from build123d import *

# Parameters (mm, degrees)
F1_DEPTH = 63.5
F2_DEPTH = 25.4
F3_DEPTH = 7.9375


with BuildPart() as f1:
    # F0 (on Front) → F1 (new body, symmetric)
    with BuildSketch(Plane.XZ):
        Polygon((22.225, 9.525), (-41.275, 9.525), (-41.275, -9.525), (41.275, -9.525), (41.275, 9.525), align=None)
    extrude(amount=F1_DEPTH, both=True)

    # F0 (on Front) → F2 (join, symmetric)
    with BuildSketch(Plane.XZ):
        with BuildLine():
            Line((22.225, 27.0002), (22.225, 9.525))
            Line((22.225, 9.525), (41.275, 9.525))
            Line((41.275, 9.525), (41.275, 27.0002))
            ThreePointArc((41.275, 27.0002), (45.92468, 38.22552), (57.15, 42.8752))
            Line((57.15, 42.8752), (67.710114, 42.8752))
            Line((67.710114, 42.8752), (67.710114, 61.9252))
            Line((67.710114, 61.9252), (57.15, 61.9252))
            add(Edge.make_bspline(
                [(56.676443, 61.921989), (56.834171, 61.923134), (56.992024, 61.924204), (57.15, 61.9252)],
                knots=[111.196311, 111.196311, 111.196311, 111.196311, 111.504536, 111.504536, 111.504536, 111.504536], degree=3))
            ThreePointArc((56.676443, 61.921989), (32.287432, 51.527905), (22.225, 27.0002))
        make_face()
    extrude(amount=F2_DEPTH, both=True)

    # F0 (on Front) → F3 (join, symmetric)
    with BuildSketch(Plane.XZ):
        with BuildLine():
            add(Edge.make_bspline(
                [(-41.275, 9.525), (-40.923248, 51.417116), (-0.225928, 61.509118), (56.676443, 61.921989)],
                knots=[0, 0, 0, 0, 111.196311, 111.196311, 111.196311, 111.196311], degree=3))
            Line((-41.275, 9.525), (22.225, 9.525))
            Line((22.225, 9.525), (22.225, 27.0002))
            ThreePointArc((22.225, 27.0002), (32.287432, 51.527905), (56.676443, 61.921989))
        make_face()
    extrude(amount=F3_DEPTH, both=True)


solid = f1.part
Source: CAD feature listing. Evaluate the final solid. Frame: model axes, mm. A direction names the side the tool comes from. Give positions to 0.01 mm unless a question says otherwise; leave off trailing zeros. Write each loop counter-clockwise with the first axis right and the second up, starting at its lowest first coordinate (ties: lowest second). Pieces come first, ordered by that corner, then holes. Notation, with made-up numbers: M -30.75,62 L 25.25,62 A24 ccw 25.25,88 Z; hole C 63,48.5 d10. An arc over 180 degrees is marked long. Return JSON: item names as keys, results as strings. Group by question number.
1) Material intervals for line 1 along Y through (x, z) = (-23.5, 31); line 2 along Y through (x, z) = (37, 46); line 3 along X through (y, z) = (-14, -4.5) (3 decimals), sorted ascending. Write a range as [from, to].
2) Set-up query: faces 1 (the face through (22.225, -17, 18)), 2 (the face through (40, -25.4, 36)), 3 (the face through (41.275, -1, 4)). Return all of +Z, -Z, +X, -X, +Y, -Y with unobstructed straight access to the full face (end or side cutting, diameter ignored); none if empty.
3) Cut plane B-B, the plane z = -3.5. Output: boundary loops of the cut face in (x, y) (3 decimals).
4) Cut plane A-A, the plane y = -38.5. Output: boundary loops of the cut face in (x, z) (3 decimals), plus the area to 3 significant figures.
5) Pin query (flat end, axial travel): P1, Ø5, axis at x = -29, y = -30.5, coming from the +Z side (3 decimals); P2, Ø1, axis at x = 25.5, z = 51, coming from the +Y side; P3, Ø5, axis at y = -12.5, z = 15.5, coming from the -X side (3 decimals); P4, Ø19, axis at y = 14, z = 14.5, coming from the -X side (3 decimals). Return the tip coordinate at first contact, or that it passes through.
Recorded:
{
 "1": {"line 1": "y = [-7.94, 7.94]", "line 2": "y = [-25.4, 25.4]", "line 3": "x = [-41.275, 41.275]"},
 "2": {"face 1": "+Z, -X, -Y", "face 2": "+Z, +X, -X, -Y", "face 3": "-Z, +X, +Y, -Y"},
 "3": {"outline": "M -41.275,-63.5 L 41.275,-63.5 L 41.275,63.5 L -41.275,63.5 Z"},
 "4": {"outline": "M -41.275,-9.525 L 41.275,-9.525 L 41.275,9.525 L -41.275,9.525 Z", "area": "1,570 mm²"},
 "5": {"P1": "stops at z = 9.525", "P2": "stops at y = 7.94", "P3": "stops at x = 22.225", "P4": "stops at x = -41.275"}
}
